Model file for the job. Use its own axes, mm. Round coordinates to 2 decimals unless told otherwise and drop trailing zeros. Order: outer loops, then holes, each group sorted by start corner. A loop starts at its lowest first (then second) coordinate and runs counter-clockwise, first axis right, second up. Notation, with made-up numbers: (68.5, 30) -> (122.5, 30) arc R16 ccw to (122.5, 41) -> close; hole circle Ø11 at (19, 69.5). An arc over 180 degrees is marked (long way). Answer as CSV lines item,"result".
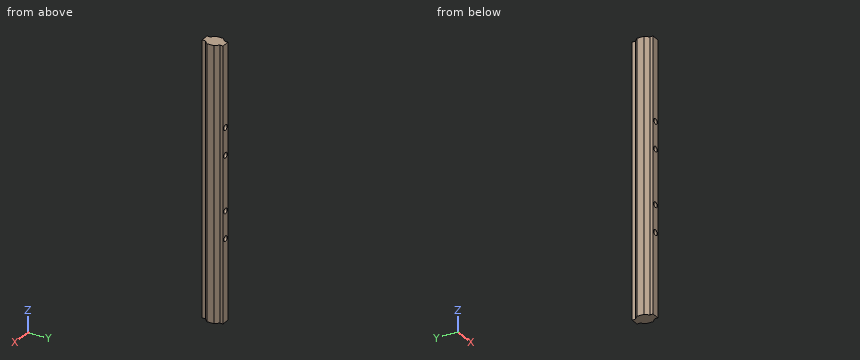
```python
from build123d import *

# Parameters (mm, degrees)
BOSS_EXTRUDE1_DEPTH = 200
SKETCH4_R           = 2
CUT_EXTRUDE1_DEPTH  = 40


with BuildPart() as part:
    # Sketch1 → Boss-Extrude1 (new body)
    with BuildSketch(Plane.XY.offset(116.106580091)):
        Polygon((-39.550290087, 5.294235639), (-36.889629915, 7.954895811), (-36.889629915, 10.362002592), (-31.010950259, 10.362002592), (-31.010950259, 7.954895811), (-28.350290087, 5.294235639), (-28.350290087, 0.029769545), (-31.010950259, -2.630890626), (-31.010950259, -5.037997408), (-36.889629915, -5.037997408), (-36.889629915, -2.630890626), (-39.550290087, 0.029769545), align=None)
    extrude(amount=BOSS_EXTRUDE1_DEPTH)

    # Sketch4 → Cut-Extrude1 (cut)
    with BuildSketch(Plane(origin=(0, -5.037997408, 0), x_dir=(-1, 0, 0), z_dir=(0, -1, 0))):
        with Locations(Location((33.950290087, -176.106580091, 0), (0, 0, 180))):
            Circle(SKETCH4_R)
        with Locations(Location((33.950290087, -196.106580091, 0), (0, 0, 180))):
            Circle(SKETCH4_R)
        with Locations(Location((33.950290087, -236.106580091, 0), (0, 0, 90))):
            Circle(SKETCH4_R)
        with Locations(Location((33.950290087, -256.106580091, 0), (0, 0, 90))):
            Circle(SKETCH4_R)
    extrude(amount=-CUT_EXTRUDE1_DEPTH, mode=Mode.SUBTRACT)


solid = part.part
```
Q1. Saw through at A-A (z = 187). Write the cut outline in (x, y).
Checks:
outline,"(-39.55, 0.03) -> (-36.89, -2.63) -> (-36.89, -5.04) -> (-31.01, -5.04) -> (-31.01, -2.63) -> (-28.35, 0.03) -> (-28.35, 5.29) -> (-31.01, 7.95) -> (-31.01, 10.36) -> (-36.89, 10.36) -> (-36.89, 7.95) -> (-39.55, 5.29) -> close"
Q2. Wall check: L1, parallel to Z at x = -34, y = -0.25; L2, parallel to Z at x = -35.75, y = 2.75; L3, parallel to X at y = -3.5, z = 237. Give the ranges that are in metal, low to high. Write a range as [from, to].
Checks:
L1,"[116.11, 174.11], [178.11, 194.11], [198.11, 234.11], [238.11, 254.11], [258.11, 316.11]"
L2,"[116.11, 175.23], [176.98, 195.23], [196.98, 235.23], [236.98, 255.23], [256.98, 316.11]"
L3,"[-36.89, -35.74], [-32.16, -31.01]"
Q3. Flat gauge pins, fed straight in: pin 1 (0.7 mm diameter, centred on y = 9.5, z = 212, fed in from +X); pin 2 (6.5 mm diameter, centred on x = -33.95, z = 196.11, fed in from +Y); pin 3 (1.9 mm diameter, centred on y = -3.5, z = 238, fed in from -X); pin 4 (4 mm diameter, centred on y = 8, z = 285, fed in from +X). Where does each tip first touch, or does it go through?
Checks:
pin 1,"x = -31.01"
pin 2,"y = 10.36"
pin 3,"x = -36.97"
pin 4,"x = -29.06"
Q4. Saw through at B-B (y = 3). Write the cut outline in (x, z), plus the area to 3 significant figures.
Checks:
outline,"(-39.55, 116.11) -> (-28.35, 116.11) -> (-28.35, 316.11) -> (-39.55, 316.11) -> close; hole circle Ø4 at (-33.95, 176.11); hole circle Ø4 at (-33.95, 196.11); hole circle Ø4 at (-33.95, 236.11); hole circle Ø4 at (-33.95, 256.11)"
area,"2,190 mm²"
